Autodesk Inventor part; units mm, degrees
ref_plane "YZ Plane" through (0, 0, 0) normal (1, 0, 0) x (0, 1, 0)
ref_plane "XZ Plane" through (0, 0, 0) normal (0, 1, 0) x (-1, 0, 0)
ref_plane "XY Plane" through (0, 0, 0) normal (0, 0, 1) x (1, 0, 0)
sketch "スケッチ1" plane through (0, 0, 0) normal (1, 0, 0) x (0, 1, 0)
  line L0 (8.9, -3) -> (8.9, -9)
  line L1 (8.9, -9) -> (8, -9)
  line L2 (8, -9) -> (8, -31)
  line L3 (8, -31) -> (0, -31)
  line L4 (0, -31) -> (0, 0)
  line L5 (8.9, -3) -> (7.7, -3)
  line L6 (7.7, -3) -> (7.7, 0)
  line L7 (7.7, 0) -> (0, 0)
  dimension "d0" = 8.9
  dimension "d1" = 3
  dimension "d2" = 9
  dimension "d3" = 31
  dimension "d4" = 7.7
  dimension "d5" = 8
revolve "回転1" add sketch "スケッチ1" angle 360 about axis through (0, 0, -31) along (0, 0, 1)
chamfer "面取り1" distance 0.2 angle 45 1 edges at (0, -7.7, 0)
properties part number "AP6MS54G" material "ABS プラスチック"
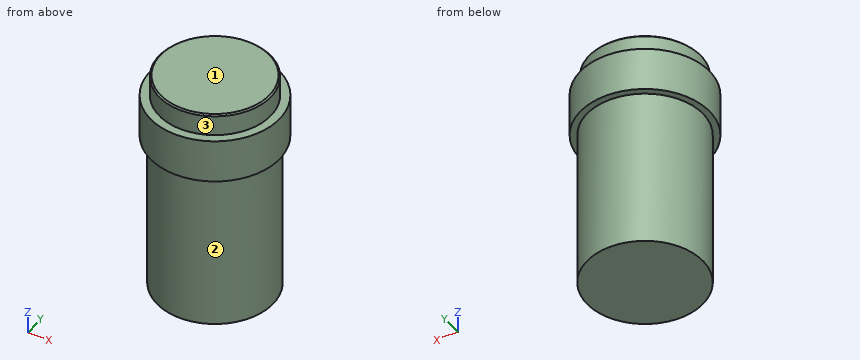
Geometry: final body of the model. Coordinates: model frame, mm. Face numbers are marked on the shaded views. A direction names the side the tool comes from. Round coordinates to 2 decimals unless told otherwise and drop trailing zeros. Order: outer loops, then holes, each group sorted by start corner. A loop starts at its lowest first (then second) coordinate and runs counter-clockwise, first axis right, second up. Notation, with made-up numbers: M 74.5,60.25 L 83.5,60.25 A29 cw 83.5,82.25 Z; hole C -1,82 d6. An arc over 180 degrees is marked long. One line per item, written item: value.
(1) Cut plane C-C (z = -6). Return the cut outline in (x, y).
Result sheet:
outline: C 0,0 d17.8
(2) Line query: probe 1 along Z at (x, y) = (-0.5, 7.75); probe 2 along Z at (x, y) = (-7.25, -5); probe 3 along Y at (x, z) = (0.25, -7). Output: solid intervals per line, ascending. Write a range as [from, to].
Result sheet:
probe 1: [-31, -3]
probe 2: [-9, -3]
probe 3: [-8.9, 8.9]
(3) Reachability of the marked faces 1, 2 and 3 from +Z, -Z, +X, -X, +Y, -Y: full face, straight path, thin tool, end or side. Return the list, or none.
Result sheet:
face 1: +Z, +X, -X, +Y, -Y
face 2: -Z
face 3: +Z
(4) Cut plane D-D (z = -15). Return the cut outline in (x, y), and give its area (3 significant figures).
Result sheet:
outline: C 0,0 d16
area: 201 mm2
(5) Pin query (flat end, axial travel): P1, Ø6, axis at x = -5, z = -5, coming from the -Y side; P2, Ø8, axis at y = -0.5, z = -10.5, coming from the -X side; P3, Ø3, axis at x = -5, z = -16, coming from the +Y side. Return the tip coordinate at first contact, or that it passes through.
Result sheet:
P1: y = -8.67
P2: x = -8.9
P3: y = 7.19
(6) Cut plane A-A (x = 0). Return the cut outline in (y, z), and give its area (3 significant figures).
Result sheet:
outline: M -8.9,-9 L -8,-9 L -8,-31 L 8,-31 L 8,-9 L 8.9,-9 L 8.9,-3 L 7.7,-3 L 7.7,-0.2 L 7.5,0 L -7.5,0 L -7.7,-0.2 L -7.7,-3 L -8.9,-3 Z
area: 505 mm2
